Geometry: final body of the model. Coordinates: model frame, mm. Round coordinates to 2 decimals unless told otherwise and drop trailing zeros. Order: outer loops, then holes, each group sorted by start corner. A loop starts at its lowest first (then second) coordinate and runs counter-clockwise, first axis right, second up. Notation, with made-up numbers: M 30.5,22.5 L 70.5,22.5 A19 cw 70.5,51.5 Z; hole C 8,58 d6. An arc over 180 degrees is marked long. Return JSON: item names as keys, results as strings. Group by question number.
Q1. Cut plane C-C on x = -0.5. Output: boundary loops of the cut face in (y, z), and give its area (3 significant figures).
Q2. Cut plane A-A on y = 2. Output: boundary loops of the cut face in (x, z).
Q3. Cut plane D-D on y = -0.25. Output: boundary loops of the cut face in (x, z).
Q4. Cut plane B-B on z = -0.65. Output: boundary loops of the cut face in (x, y), and give its area (3 significant figures).
Q5. Ray query, probe 1 along Y at (x, z) = (-0.45, -0.05); probe 2 along Z at (x, y) = (0.1, -2); probe 3 along Y at (x, z) = (-0.05, 0.25). Return the intervals inside material, ascending.
Q6. Contact query for flat-ended pins moving along their axis: pin 1 (0.5 mm diameter, centred on x = 0, y = 3.5, fed in from -Z); pin 2 (0.7 mm diameter, centred on y = 3.5, z = 0, fed in from -X). Output: stop coordinate, or through.
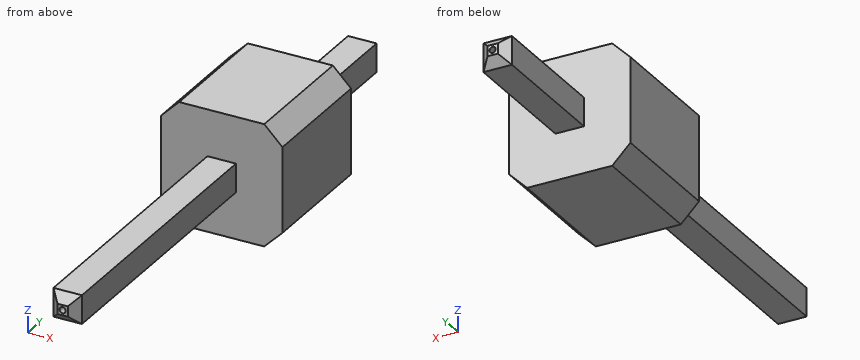
Autodesk Inventor part; units mm, degrees
ref_plane "YZ Plane" through (0, 0, 0) normal (1, 0, 0) x (0, 1, 0)
ref_plane "XZ Plane" through (0, 0, 0) normal (0, 1, 0) x (-1, 0, 0)
ref_plane "XY Plane" through (0, 0, 0) normal (0, 0, 1) x (1, 0, 0)
sketch "Sketch1" plane through (0, 0, 0) normal (0, 1, 0) x (-1, 0, 0)
  line L0 (-1.27, 1.27) -> (1.27, 1.27)
  line L1 (1.27, 1.27) -> (1.27, -1.27)
  line L2 (1.27, -1.27) -> (-1.27, -1.27)
  line L3 (-1.27, -1.27) -> (-1.27, 1.27)
  line L4 (-1.27, 1.27) -> (1.27, -1.27) construction
  line L5 (1.27, 1.27) -> (-1.27, -1.27) construction
  point P0 (0, 0)
  dimension "d0" = 2.54
extrude "Extrusion1" add sketch "Sketch1" along normal blind 2.6035
chamfer "Chamfer1" distance 0.381 angle 45 4 edges at (1.27, 1.3017, 1.27) (-1.27, 1.3017, 1.27) (1.27, 1.3017, -1.27) (-1.27, 1.3017, -1.27)
sketch "Sketch2" plane through (0, 2.6035, 0) normal (0, 1, 0) x (1, 0, 0)
  line L0 (0.2984, 0.2984) -> (-0.2984, 0.2984)
  line L1 (-0.2984, 0.2984) -> (-0.2984, -0.2984)
  line L2 (-0.2984, -0.2984) -> (0.2984, -0.2984)
  line L3 (0.2984, -0.2984) -> (0.2984, 0.2984)
  line L4 (0.2984, 0.2984) -> (-0.2984, -0.2984) construction
  line L5 (-0.2984, 0.2984) -> (0.2984, -0.2984) construction
  point P0 (0, 0)
  dimension "d6" = 0.5969
extrude "Extrusion2" add sketch "Sketch2" along normal blind 2.921 and the other way blind 8.636
chamfer "Chamfer2" distance 0.1905 angle 45 8 edges at (0.2984, 5.5245, 0) (0, 5.5245, -0.2984) (-0.2984, 5.5245, 0) (0, 5.5245, 0.2984) (0, -6.0325, -0.2984) (0.2984, -6.0325, 0) (0, -6.0325, 0.2984) (-0.2984, -6.0325, 0)
sketch "Sketch3" plane through (0, 5.5245, 0) normal (0, 1, 0) x (1, 0, 0)
  circle A0 centre (0, 0) radius 0.0635
  dimension "d14" = 0.127
extrude "Extrusion3" cut sketch "Sketch3" against normal through all
properties part number "Single Short Male Header"
Result sheet:
{
 "1": {"outline": "M 0,-1.27 L 2.6,-1.27 L 2.6,1.27 L 0,1.27 Z", "area": "6.61 mm²"},
 "2": {"outline": "M -1.27,-0.89 L -0.89,-1.27 L 0.89,-1.27 L 1.27,-0.89 L 1.27,0.89 L 0.89,1.27 L -0.89,1.27 L -1.27,0.89 Z; hole C 0,0 d0.13"},
 "3": {"outline": "M -0.3,-0.3 L 0.3,-0.3 L 0.3,0.3 L -0.3,0.3 Z; hole C 0,0 d0.13"},
 "4": {"outline": "M -1.27,0 L 1.27,0 L 1.27,2.6 L -1.27,2.6 Z", "area": "6.61 mm²"},
 "5": {"probe 1": "y = 0 to 2.6", "probe 2": "z = -0.3 to 0.3", "probe 3": "y = -5.89 to 5.38"},
 "6": {"pin 1": "stops at z = -0.3", "pin 2": "stops at x = -0.3"}
}
